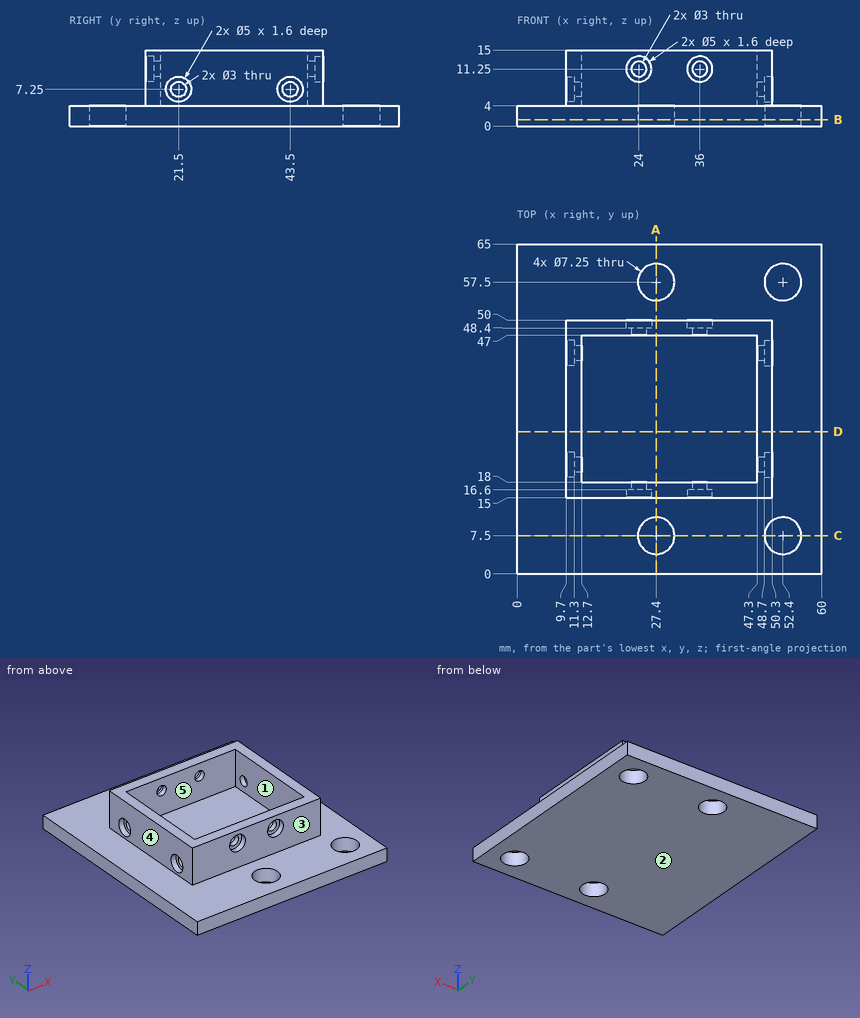
The figure shows three views and two pictorial views of one solid part (mm, origin at its lowest corner). Answer the questions. A direction names the side the tool comes from. Round coordinates to 2 decimals unless told otherwise and drop trailing zeros. Order: outer loops, then holes, each group sorted by start corner. A loop starts at its lowest first (then second) coordinate and runs counter-clockwise, first axis right, second up. Notation, with made-up numbers: (53, -2.75) - (94, -2.75) arc R14 ccw to (94, 5.25) - close; hole circle Ø1 at (77.5, 76.25). An arc over 180 degrees is marked (long way). Write item = value, one per line. Start each with the question number.
1) Section D-D, the plane y = 28 is taken. Write down the section's boundary in (x, z).
2) Given pin 1 (4.5 mm diameter, centred on y = 21.5, z = 7.25, fed in from +X); pin 2 (1.5 mm diameter, centred on x = 21, y = 26, fed in from +Z); pin 3 (5 mm diameter, centred on x = 10, z = 13.5, fed in from +Y), each flat-ended and moving along its own axis, determine where each tip first touches the part or whether it passes through.
3) Straight lines are drawn through the part: L1, parallel to Y at x = 10.3, z = 7.25; L2, parallel to Y at x = 39, z = 9.25; L3, parallel to Z at x = 36, y = 48. For each, find the intervals that lie inside material, in ascending order.
4) For a pull along Y with two mould halves and no side action, classify the marked faces 3, 4 and 5 as released by +Y, released by -Y, zero draft, split by the parting line, or undercut.
5) Section C-C, the plane y = 7.5 is taken. Write down the section's boundary in (x, z) (3 decimals), plus the area to 3 significant figures.
6) Section A-A, the plane x = 27.4 is taken. Write down the section's boundary in (y, z) (3 decimals).
7) Section B-B, the plane z = 1.25 is taken. Write down the section's boundary in (x, y) (3 decimals).
8) For the marked faces 1 and 2, determine the directions among +Z, -Z, +X, -X, +Y, -Y from which every point of the face is accessible in a straight line to the end or side of a thin tool.
Results list:
q1.outline = (0, 0) - (60, 0) - (60, 4) - (50.3, 4) - (50.3, 15) - (47.3, 15) - (47.3, 4) - (12.7, 4) - (12.7, 15) - (9.7, 15) - (9.7, 4) - (0, 4) - close
q2.pin_1 = 48.7
q2.pin_2 = 4
q2.pin_3 = 50
q3.L1 = 15 to 19, 24 to 41, 46 to 50
q3.L2 = 15 to 18, 47 to 50
q3.L3 = 0 to 9.75, 12.75 to 15
q4.face_3 = released by -Y
q4.face_4 = zero draft
q4.face_5 = undercut
q5.outline = (0, 0) - (23.775, 0) - (23.775, 4) - (0, 4) - close; (31.025, 0) - (48.775, 0) - (48.775, 4) - (31.025, 4) - close; (56.025, 0) - (60, 0) - (60, 4) - (56.025, 4) - close
q5.area = 182 mm^2
q6.outline = (0, 0) - (3.875, 0) - (3.875, 4) - (0, 4) - close; (11.125, 0) - (53.875, 0) - (53.875, 4) - (50, 4) - (50, 15) - (47, 15) - (47, 4) - (18, 4) - (18, 15) - (15, 15) - (15, 4) - (11.125, 4) - close; (61.125, 0) - (65, 0) - (65, 4) - (61.125, 4) - close
q7.outline = (0, 0) - (60, 0) - (60, 65) - (0, 65) - close; hole circle Ø7.25 at (27.4, 7.5); hole circle Ø7.25 at (27.4, 57.5); hole circle Ø7.25 at (52.4, 7.5); hole circle Ø7.25 at (52.4, 57.5)
q8.face_1 = +Z
q8.face_2 = -Z, +X, -X, +Y, -Y
